from build123d import *

# Parameters (mm, degrees)
BOSS_EXTRUDE1_DEPTH     = 18.915
CUT_EXTRUDE1_DEPTH      = 73.981798073
CUT_EXTRUDE1_DEPTH_BACK = 73.981798073
SKETCH42_R              = 3.3
SKETCH42_R_2            = 3.5


with BuildPart() as part:
    # Sketch41 → Boss-Extrude1 (new, symmetric)
    with BuildSketch(Plane(origin=(0, 0, 0), x_dir=(0, 0, -1), z_dir=(1, 0, 0))):
        Polygon((4.025167823, -62.9), (17.5, -62.9), (17.5, -67.9), (-18.925, -67.9), (-18.925, 0), (2.88943812, 0), (2.88943812, -19.25), (-3.46056188, -19.25), (-3.46056188, -37.9), (4.025167823, -37.9), align=None)
    extrude(amount=BOSS_EXTRUDE1_DEPTH, both=True)

    # Sketch42 → Cut-Extrude1 (cut, two sides: drawn at the far end of the back side and taken through both)
    with BuildSketch(Plane.XY.offset(-CUT_EXTRUDE1_DEPTH_BACK)):
        with Locations((0, -10.5)):
            Circle(SKETCH42_R)
        with Locations((0, -50.4)):
            Circle(SKETCH42_R_2)
        with Locations((-8.501076983, -28.575)):
            Circle(SKETCH42_R)
        with Locations((9.298923017, -28.575)):
            Circle(SKETCH42_R)
    extrude(amount=CUT_EXTRUDE1_DEPTH + CUT_EXTRUDE1_DEPTH_BACK, mode=Mode.SUBTRACT)


solid = part.part
Input: part model. Units: mm. Frame: model coordinates. A direction names the side the tool comes from. Coordinates: 2 decimals unless noted, no trailing zeros. Order: outer loops, then holes, each group sorted by start corner. A loop starts at its lowest first (then second) coordinate and runs counter-clockwise, first axis right, second up. Notation, with made-up numbers: M 67.5,66 L 120.5,66 A16 cw 120.5,89 Z; hole C 14,-24.75 d5. An arc over 180 degrees is marked long. Write item = value, one per line. Start each with the question number.
(1) Section A-A on x = 0. Output: boundary loops of the cut face in (y, z) (3 decimals), and give its area (3 significant figures).
(2) Section B-B on z = 2. Output: boundary loops of the cut face in (x, y) (3 decimals).
(3) Pull-direction query (X, two-part tool) for faces 4 (the cylindrical face through (-5.353, -27.584, 11.085)), 5 (the flat face through (0, -62.9, -11)), 6 (the flat face through (18.915, -33, 9)); classes: released by +X, released by -X, zero draft, split by the parting line, or undercut.
(4) Section C-C on y = -10.5. Output: boundary loops of the cut face in (x, z) (3 decimals), and give its area (3 significant figures).
(5) First-contact query: P1, Ø9.5, axis at x = 2.5, y = -25, coming from the -Z side; P2, Ø8.5, axis at x = 0, y = -10.5, coming from the -Z side; P3, Ø6.5, axis at x = -7.5, z = -10.5, coming from the +Y side. Flat tips, straight axial feed; report the tip coordinate or a pass-through.
(6) Section D-D on x = -7. Output: boundary loops of the cut face in (y, z) (3 decimals).
(7) Line query: line 1 along Y through (x, z) = (0, 12.5); line 2 along X through (y, z) = (-50.4, 4) (3 decimals); line 3 along X through (y, z) = (-27, 11) (3 decimals). Output: solid intervals per line, ascending. Write a range as [from, to].
(8) Reachability of faces 1 (the flat face through (4, -9, -2.889)), 2 (the flat face through (0, -28, 3.461)), 3 (the cylindrical face through (6.87, -26.34, 11.08)) from +Z, -Z, +X, -X, +Y, -Y: full face, straight path, thin tool, end or side. Return the list, or none.
Result set:
q1.outline = M -67.9,-17.5 L -62.9,-17.5 L -62.9,-4.025 L -53.9,-4.025 L -53.9,18.925 L -67.9,18.925 Z; M -46.9,-4.025 L -37.9,-4.025 L -37.9,3.461 L -19.25,3.461 L -19.25,-2.889 L -13.8,-2.889 L -13.8,18.925 L -46.9,18.925 Z; M -7.2,-2.889 L 0,-2.889 L 0,18.925 L -7.2,18.925 Z
q1.area = 1,160 mm²
q2.outline = M -18.915,-67.9 L 18.915,-67.9 L 18.915,-37.9 L -18.915,-37.9 Z; M -18.915,-19.25 L 18.915,-19.25 L 18.915,0 L -18.915,0 Z; hole C 0,-50.4 d7; hole C 0,-10.5 d6.6
q3.face_4 = undercut
q3.face_5 = zero draft
q3.face_6 = released by +X
q4.outline = M -18.915,-2.889 L -3.3,-2.889 L -3.3,18.925 L -18.915,18.925 Z; M 3.3,-2.889 L 18.915,-2.889 L 18.915,18.925 L 3.3,18.925 Z
q4.area = 681 mm²
q5.P1 = 3.46
q5.P2 = -2.89
q5.P3 = -62.9
q6.outline = M -67.9,-17.5 L -62.9,-17.5 L -62.9,-4.025 L -37.9,-4.025 L -37.9,3.461 L -31.514,3.461 L -31.514,18.925 L -67.9,18.925 Z; M -25.636,3.461 L -19.25,3.461 L -19.25,-2.889 L 0,-2.889 L 0,18.925 L -25.636,18.925 Z
q7.line_1 = [-67.9, -53.9], [-46.9, -13.8], [-7.2, 0]
q7.line_2 = [-18.915, -3.5], [3.5, 18.915]
q7.line_3 = [-18.915, -11.401], [-5.601, 6.399], [12.199, 18.915]
q8.face_1 = -Z, +X, -X, +Y
q8.face_2 = -Z, +X, -X
q8.face_3 = +Z, -Z
